Print and shaded views of the part. All mm, measured from the part's lowest x, y and z. A direction names the side the tool comes from. Coordinates: 2 decimals unless noted, no trailing zeros. Loops run counter-clockwise (first coordinate to the right, second up) from the corner with the lowest first, then second, coordinate; pieces in that order, holes last. Notation, with made-up numbers: (-33, 53) -> (2, 53) arc R20 ccw to (2, 76) -> close; hole circle Ø2 at (43.25, -23.75). An arc over 180 degrees is marked (long way). One line per question, with ' | ' between items. Start each with the question number.
1) Cut at B-B (z = 484.5). List the corners of the cut face in (x, y), plus the area to 3 significant figures.
2) 3-axis set-ups, long thin cutter, end or side, ignore diameter. For the marked faces 5, 6 and 7: which of +Z, -Z, +X, -X, +Y, -Y reach the whole face in a straight line?
3) Cut at C-C (y = 458.5). List the corners of the cut face in (x, z), plus the area to 3 significant figures.
4) Cut at A-A (x = 55.5). List the corners of the cut face in (y, z).
5) Probe L1, parallel to Z at x = 116.5, y = 44; L2, parallel to X at y = 63, z = 194.5; L3, parallel to Z at x = 10, y = 253. List the from-to ranges inside material, lowest first. Write a range as from..to.
6) Two-plate mould, pull along X, no slides. Class the marked faces 1, 2, 3 and 4: released by +X, released by -X, zero draft, split by the parting line, or undercut.
7) Drop flat-ended pins along their axis: pin 1 (10 mm diameter, centred on x = 129.5, z = 227, fed in from +Y); pin 2 (10 mm diameter, centred on x = 63.5, z = 103, fed in from -Y); pin 3 (1 mm diameter, centred on y = 68.5, z = 434.5, fed in from -X). Give the stop position or say it passes through.
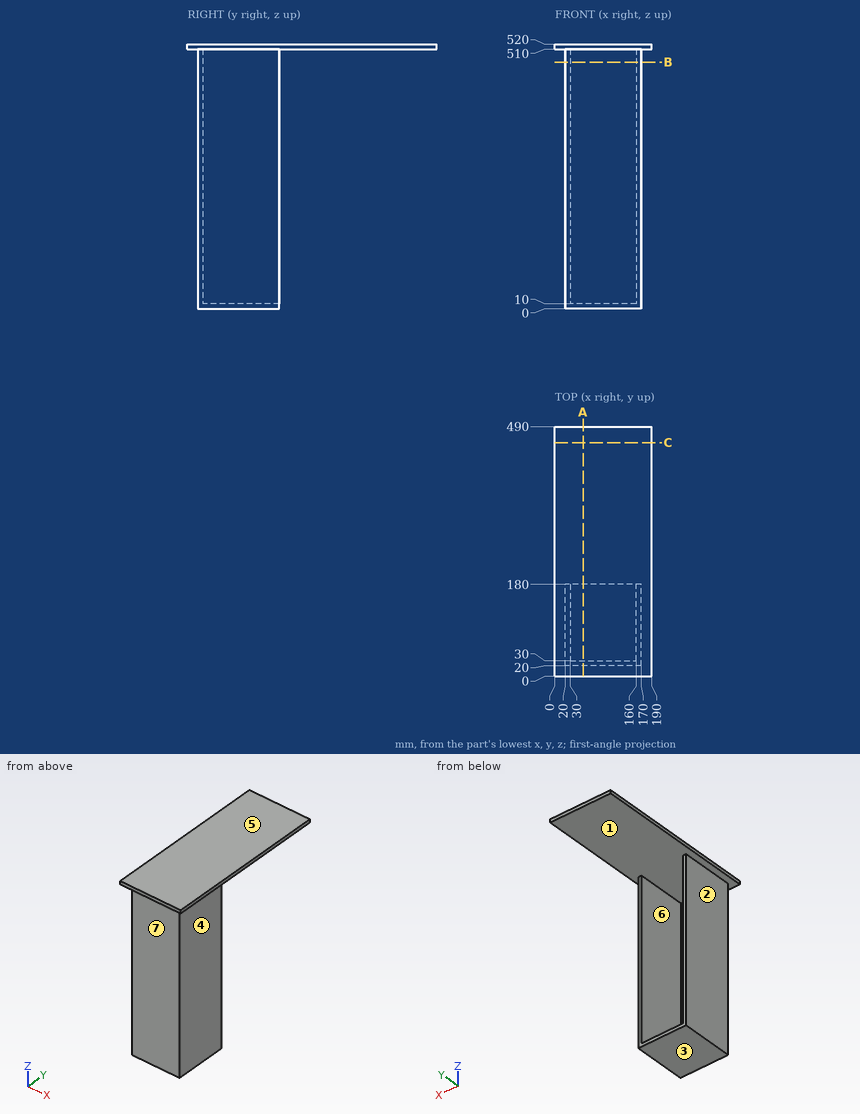
Reported:
1) outline: (20, 20) -> (170, 20) -> (170, 180) -> (160, 180) -> (160, 30) -> (30, 30) -> (30, 180) -> (20, 180) -> close | area: 4,500 mm²
2) face 5: +Z, +X, -X, +Y, -Y | face 6: +Y | face 7: -Z, +X, -X, -Y
3) outline: (0, 510) -> (190, 510) -> (190, 520) -> (0, 520) -> close | area: 1,900 mm²
4) outline: (0, 510) -> (20, 510) -> (20, 0) -> (180, 0) -> (180, 10) -> (30, 10) -> (30, 510) -> (490, 510) -> (490, 520) -> (0, 520) -> close
5) L1: z = 0..10, 510..520 | L2: x = 20..30, 160..170 | L3: z = 510..520
6) face 1: undercut | face 2: released by -X | face 3: zero draft | face 4: released by +X
7) pin 1: stops at y = 30 | pin 2: stops at y = 20 | pin 3: stops at x = 20
